from build123d import *

# Parameters (mm, degrees)
SKETCH1_W                = 30
SKETCH1_H                = 18
BOSS_EXTRUDE1_DEPTH      = 19
BOSS_EXTRUDE2_DEPTH      = 19
BOSS_EXTRUDE2_DEPTH_BACK = 37
SKETCH2_R                = 3.5
FILLET1_R                = 2


with BuildPart() as part:
    # Sketch1 → Boss-Extrude1 (new body)
    with BuildSketch(Plane(origin=(0, 0, 0), x_dir=(1, 0, 0), z_dir=(0, 1, 0))):
        Rectangle(SKETCH1_W, SKETCH1_H)
    extrude(amount=BOSS_EXTRUDE1_DEPTH)

    # Sketch2 → Boss-Extrude2 (add, two sides: drawn at the far end of the back side and taken through both)
    with BuildSketch(Plane(origin=(15, 0, 0), x_dir=(0, 0, -1), z_dir=(1, 0, 0)).offset(-BOSS_EXTRUDE2_DEPTH_BACK)):
        with Locations((0, 9.5)):
            Circle(SKETCH2_R)
    extrude(amount=BOSS_EXTRUDE2_DEPTH + BOSS_EXTRUDE2_DEPTH_BACK)

    # Fillet1
    fillet1_edges = [part.edges().sort_by_distance(p)[0] for p in [
        (0, 19, 9),
        (0, 0, 9),
        (0, 0, -9),
        (0, 19, -9),
    ]]
    fillet(fillet1_edges, radius=FILLET1_R)


solid = part.part
Input: part model. Units: mm. Frame: model coordinates. A direction names the side the tool comes from. Give positions to 0.01 mm unless a question says otherwise; leave off trailing zeros. Order: outer loops, then holes, each group sorted by start corner. A loop starts at its lowest first (then second) coordinate and runs counter-clockwise, first axis right, second up. Notation, with made-up numbers: (2, 53.5) - (57, 53.5) arc R33 cw to (57, 81.5) - close; hole circle Ø10 at (-35.75, 41). An arc over 180 degrees is marked (long way). Answer as a JSON object with one key per item and string values. Group by question number.
Q1. Cut plane A-A, the plane z = 0. Output: boundary loops of the cut face in (x, y), then the cut area to 3 significant figures.
Q2. Cut plane C-C, the plane x = -15.5. Output: boundary loops of the cut face in (y, z).
Q3. Cut plane D-D, the plane y = 4.75. Output: boundary loops of the cut face in (x, z), then the cut area to 3 significant figures.
Q4. Set-up query: faces 1 (the face through (-18.549, 6.083, 0.759)), 2 (the face through (0, 9, -9)), 3 (the face through (15, 9, 4)). Return all of +Z, -Z, +X, -X, +Y, -Y with unobstructed straight access to the full face (end or side cutting, diameter ignored); none if empty.
Q5. Cut plane B-B, the plane y = 9.5. Output: boundary loops of the cut face in (x, z), then the cut area to 3 significant figures.
Q6. Line query: probe 1 along X at (y, z) = (4, 4.5); probe 2 along Z at (x, y) = (-19.5, 10.25); probe 3 along Y at (x, z) = (6, 7.5). Output: solid intervals per line, ascending.
Q7. First-contact query: pin 1 Ø3 at (x, z) = (26.5, 1.5) entering from -Y. Flat tip, straight axial feed; report the tip coordinate or a pass-through.
Results:
{
 "1": {"outline": "(-22, 6) - (-15, 6) - (-15, 0) - (15, 0) - (15, 6) - (34, 6) - (34, 13) - (15, 13) - (15, 19) - (-15, 19) - (-15, 13) - (-22, 13) - close", "area": "752 mm^2"},
 "2": {"outline": "circle Ø7 at (9.5, 0)"},
 "3": {"outline": "(-15, -9) - (15, -9) - (15, 9) - (-15, 9) - close", "area": "540 mm^2"},
 "4": {"face 1": "-X", "face 2": "-Z, +X, -X, +Y, -Y", "face 3": "+X"},
 "5": {"outline": "(-22, -3.5) - (-15, -3.5) - (-15, -9) - (15, -9) - (15, -3.5) - (34, -3.5) - (34, 3.5) - (15, 3.5) - (15, 9) - (-15, 9) - (-15, 3.5) - (-22, 3.5) - close", "area": "722 mm^2"},
 "6": {"probe 1": "-15 to 15", "probe 2": "-3.42 to 3.42", "probe 3": "0.06 to 18.94"},
 "7": {"pin 1": "y = 6"}
}
